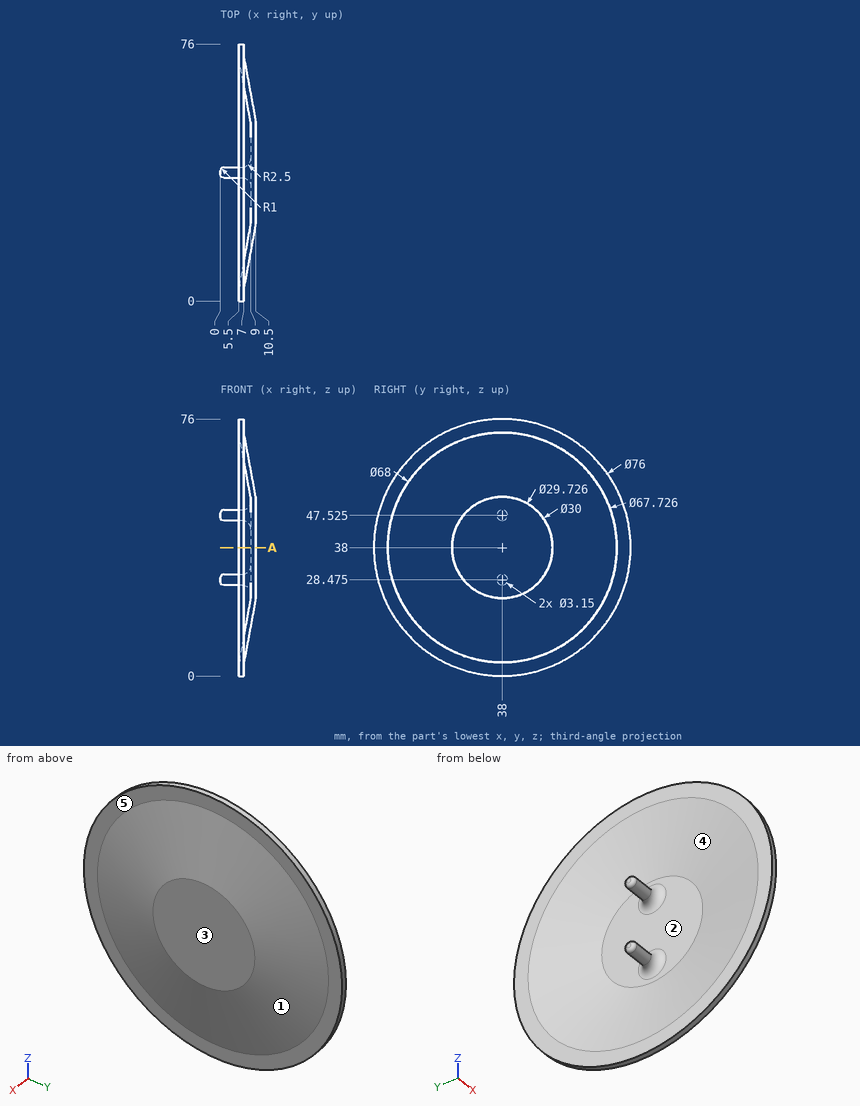
The figure shows three views and two pictorial views of one solid part (mm, origin at its lowest corner). Answer the questions. A direction names the side the tool comes from. Coordinates: 2 decimals unless noted, no trailing zeros. Write each loop counter-clockwise with the first axis right and the second up, starting at its lowest first coordinate (ties: lowest second). Pieces come first, ordered by that corner, then holes. Notation, with made-up numbers: (87, 27.25) -> (111, 27.25) arc R23 ccw to (111, 38.25) -> close; hole circle Ø9 at (11.5, -39.75). An arc over 180 degrees is marked (long way). Return JSON: item names as keys, results as strings.
(1) Which of the six approach directions +Z, -Z, +X, -X, +Y, -Y give full straight-line access (tool end or side, diameter ignored) to the marked faces 4 and 5?
Answers below:
{"face 4": "-X", "face 5": "+X"}
(2) Consider line 1 along X through (y, z) = (44.5, 33); line 2 along Y through (x, z) = (4, 28); line 3 along X through (y, z) = (65.5, 44). Determine where each line is inside the solid, lowest interval first. Write a range as from..to.
Answers below:
{"line 1": "9..10.5", "line 2": "36.5..39.5", "line 3": "6.55..8.08"}
(3) For a pull along Z with two mould halves and no side action, classify the marked faces 1, 2 and 3 as pulls with the +Z half, pulls with the -Z half, needs draft (parallel to the pull), parting line crosses it, or undercut.
Answers below:
{"face 1": "parting line crosses it", "face 2": "undercut", "face 3": "needs draft"}
(4) Each of these flat-tipped pins is pushed along its axis until it touches: P1, Ø3, axis at x = 7.5, z = 29, coming from the -Y side; P2, Ø6, axis at y = 48, z = 11.5, coming from the +X side; P3, Ø6, axis at x = 7.5, y = 14.5, coming from the -Z side. Where does it stop, or does it pass through?
Answers below:
{"P1": "y = 0.76", "P2": "x = 8.6", "P3": "z = 6.03"}
(5) The part is cut by section A-A on z = 38. Give the vertices of the cut face in (x, y), then the cut area to 3 significant figures.
Answers below:
{"outline": "(5.5, 0) -> (7, 0) -> (7, 4) -> (10.5, 23) -> (10.5, 53) -> (7, 72) -> (7, 76) -> (5.5, 76) -> (5.5, 71.86) -> (9, 52.86) -> (9, 23.14) -> (5.5, 4.14) -> close", "area": "115 mm^2"}
